Source: CAD feature listing. Evaluate the final solid. Frame: model axes, mm. A direction names the side the tool comes from. Round coordinates to 2 decimals unless told otherwise and drop trailing zeros. Loops run counter-clockwise (first coordinate to the right, second up) from the corner with the lowest first, then second, coordinate; pieces in that order, holes last. Notation, with made-up numbers: M -9,84 L 21,84 A17 cw 21,116 Z; hole C -23,20 d11. An arc over 180 degrees is marked long. Answer as a JSON object with one key per item and string values.
Autodesk Inventor part; units mm, degrees
ref_plane "YZ Plane" through (0, 0, 0) normal (1, 0, 0) x (0, 1, 0)
ref_plane "XZ Plane" through (0, 0, 0) normal (0, 1, 0) x (-1, 0, 0)
ref_plane "XY Plane" through (0, 0, 0) normal (0, 0, 1) x (1, 0, 0)
sketch "スケッチ1" plane through (0, 0, 0) normal (0, 0, 1) x (1, 0, 0)
  line L0 (0, 0) -> (30.5, 0)
  line L1 (30.5, 0) -> (30.5, 21)
  line L2 (30.5, 21) -> (0, 21)
  line L3 (0, 21) -> (0, 0)
  dimension "d0" = 30.5
  dimension "d1" = 21
extrude "プレート1" add sketch "スケッチ1" along normal blind 1.5
sketch "スケッチ2" plane through (30.5, 21, 1.5) normal (1, 0, 0) x (0, 1, 0)
  line L0 (-21, 0) -> (0, 0)
  line L1 (0, 0) -> (0, 8.5)
  line L2 (0, 8.5) -> (-21, 8.5)
  line L3 (-21, 8.5) -> (-21, 0)
edge flange "フランジ1" height 10 angle 90 thickness 1.5 bend radius 1.5 thickness toward (1, 0, 0) relief tear relief width 1.5 relief depth 0.75 corner gap 1.5 corner form 0 edges at (30.5, 10.5, 1.5) (0, 10.5, 1.5) wall of the first edge with corners at (30.5, 0, 1.5) (30.5, 21, 1.5) (30.5, 21, 10) (30.5, 0, 10)
bend "曲げ1"
corner "コーナー1"
sketch "スケッチ3" plane through (32, 0, 10) normal (1, 0, 0) x (0, 0, -1)
  line L0 (4, 0) -> (4, 21) construction
  line L1 (7, 21) -> (0, 21)
  line L2 (0, 21) -> (0, 0)
  line L3 (0, 10.5) -> (4, 10.5)
  point P0 (10, 0)
  point P1 (4, 2.5)
  point P2 (4, 18.5)
  dimension "d15" = 4
  dimension "d16" = 16
hole "穴1" at (32, 2.5, 6) at (32, 18.5, 6) direction (-1, 0, 0) diameter 2.2 end through all
sketch "スケッチ4" plane through (0, 0, 0) normal (0, 0, -1) x (-1, 0, 0)
  line L0 (-32, 0) -> (-32, 21)
  line L1 (-32, 10.5) -> (1.5, 10.5)
  line L2 (1.5, 21) -> (1.5, 0)
  line L3 (-29, 0) -> (-1.5, 0)
  line L4 (-15.25, 0) -> (-15.25, 21)
  line L5 (-1.5, 21) -> (-29, 21)
  point P0 (0, 0)
  point P1 (-23.25, 3.5)
  point P2 (-23.25, 17.5)
  point P3 (-7.25, 3.5)
  point P4 (-7.25, 17.5)
  dimension "d31" = 14
  dimension "d32" = 16
hole "穴2" at (23.25, 3.5, 0) at (23.25, 17.5, 0) at (7.25, 3.5, 0) at (7.25, 17.5, 0) direction (0, 0, 1) diameter 4.5 end through all
equation "\"d22\" = Thickness"
equation "\"d29\" = Thickness"
equation "\"d2\" = Thickness"
equation "\"d3\" = BendReliefWidth"
equation "\"d4\" = BendReliefDepth"
equation "\"d5\" = MinimumRemnant"
equation "\"d6\" = TransitionRadius"
equation "\"d9\" = BendRadius"
equation "\"d10\" = CornerReliefSize"
equation "\"d11\" = GapSize"
equation "\"d12\" = JacobiRadiusSize"
equation "\"BendRadius\" = Thickness"
equation "\"BendReliefWidth\" = Thickness"
equation "\"BendReliefDepth\" = 0.5 * Thickness"
equation "\"CornerReliefSize\" = 4 * Thickness"
equation "\"MinimumRemnant\" = 2 * Thickness"
equation "\"TransitionRadius\" = BendRadius"
equation "\"JacobiRadiusSize\" = BendRadius"
equation "\"GapSize\" = Thickness"
properties part number "servo_bracket" material "アルミニウム 6061"
Item 1: Line query: probe 1 along Y at (x, z) = (31.15, 6); probe 2 along X at (y, z) = (10.75, 9.75); probe 3 along X at (y, z) = (17.5, 0.3). Output: solid intervals per line, ascending. Write a range as from..to.
Answer sheet:
{"probe 1": "y = 0..1.4, 3.6..17.4, 19.6..21", "probe 2": "x = -1.5..0, 30.5..32", "probe 3": "x = 0.19..5, 9.5..21, 25.5..30.31"}
Item 2: Pull-direction query (Y, two-part tool) for faces 1 (the flat face through (-1, 10, 10)), 2 (the cylindrical face through (5.02, 3.21, 0.76)), 3 (the flat face through (15, 21, 1)); classes: pulls with the +Y half, pulls with the -Y half, needs draft (parallel to the pull), parting line crosses it, or undercut.
Answer sheet:
{"face 1": "needs draft", "face 2": "undercut", "face 3": "pulls with the +Y half"}
Item 3: Section B-B on z = 6. Return the cut outline in (x, y), then the cut area to 3 significant figures.
Answer sheet:
{"outline": "M -1.5,0 L 0,0 L 0,1.4 L -1.5,1.4 Z; M -1.5,3.6 L 0,3.6 L 0,17.4 L -1.5,17.4 Z; M -1.5,19.6 L 0,19.6 L 0,21 L -1.5,21 Z; M 30.5,0 L 32,0 L 32,1.4 L 30.5,1.4 Z; M 30.5,3.6 L 32,3.6 L 32,17.4 L 30.5,17.4 Z; M 30.5,19.6 L 32,19.6 L 32,21 L 30.5,21 Z", "area": "49.8 mm²"}
Item 4: Section C-C on x = 23.25. Return the cut outline in (y, z), then the cut area to 3 significant figures.
Answer sheet:
{"outline": "M 0,0 L 1.25,0 L 1.25,1.5 L 0,1.5 Z; M 5.75,0 L 15.25,0 L 15.25,1.5 L 5.75,1.5 Z; M 19.75,0 L 21,0 L 21,1.5 L 19.75,1.5 Z", "area": "18.0 mm²"}
Item 5: Section D-D on y = 18.5. Return the cut outline in (x, z).
Answer sheet:
{"outline": "M -1.5,3 A3 ccw 1.5,0 L 5.23,0 L 5.23,1.5 L 1.5,1.5 A1.5 cw 0,3 L 0,4.9 L -1.5,4.9 Z; M -1.5,7.1 L 0,7.1 L 0,10 L -1.5,10 Z; M 9.27,0 L 21.23,0 L 21.23,1.5 L 9.27,1.5 Z; M 25.27,0 L 29,0 A3 ccw 32,3 L 32,4.9 L 30.5,4.9 L 30.5,3 A1.5 cw 29,1.5 L 25.27,1.5 Z; M 30.5,7.1 L 32,7.1 L 32,10 L 30.5,10 Z"}
Item 6: Contact query for flat-ended pins moving along their axis: pin 1 Ø1.8 at (y, z) = (18.5, 6) entering from +X; pin 2 Ø6 at (x, y) = (7.25, 17.5) entering from +Z. Output: stop coordinate, or through.
Answer sheet:
{"pin 1": "passes through", "pin 2": "stops at z = 1.5"}
Item 7: Access query for faces 4 (the cylindrical face through (31.24, 2.921, 4.984)), 5 (the flat face through (15, 11, 1.5)). Directions: +Z, -Z, +X, -X, +Y, -Y. A direction counts if a zero-diameter tool reaches every point of the face in a straight line with its end or side. Return the directions, or none.
Answer sheet:
{"face 4": "+X, -X", "face 5": "+Z, +Y, -Y"}
Item 8: Section A-A on z = 9.5. Return the cut outline in (x, y), then the cut area to 3 significant figures.
Answer sheet:
{"outline": "M -1.5,0 L 0,0 L 0,21 L -1.5,21 Z; M 30.5,0 L 32,0 L 32,21 L 30.5,21 Z", "area": "63.0 mm²"}
